Autodesk Inventor part; units mm, degrees
ref_plane "YZ Plane" through (0, 0, 0) normal (1, 0, 0) x (0, 1, 0)
ref_plane "XZ Plane" through (0, 0, 0) normal (0, 1, 0) x (-1, 0, 0)
ref_plane "XY Plane" through (0, 0, 0) normal (0, 0, 1) x (1, 0, 0)
sketch "Szkic1" plane through (0, 0, 0) normal (0, 1, 0) x (-1, 0, 0)
  line L0 (0, 0) -> (-50, 0)
  line L1 (-50, 0) -> (-50, -90)
  line L2 (-50, -90) -> (0, -90)
  line L3 (0, -90) -> (0, 0)
  dimension "d0" = 50
  dimension "d1" = 90
extrude "Wyciągnięcie proste1" add sketch "Szkic1" along normal blind 20
sketch "Szkic2" plane through (0, 20, 0) normal (0, 1, 0) x (1, 0, 0)
  line L0 (50, 0) -> (50, 90)
  line L1 (50, 65) -> (30, 65)
  line L2 (30, 65) -> (30, 25)
  line L3 (30, 25) -> (50, 25)
  line L4 (50, 25) -> (50, 65)
  line L5 (50, 90) -> (0, 90)
  point P0 (0, 0)
  dimension "d4" = 20
  dimension "d5" = 40
  dimension "d6" = 25
extrude "Wyciągnięcie proste2" cut sketch "Szkic2" against normal blind 10
sketch "Szkic3" plane through (0, 10, 0) normal (0, 1, 0) x (1, 0, 0)
  line L0 (50, 65) -> (50, 25)
  circle A0 centre (50, 45) radius 10
  point P0 (0, 0)
  point P1 (50, 35)
  point P2 (50, 55)
  dimension "d9" = 20
extrude "Wyciągnięcie proste3" cut sketch "Szkic3" against normal through all contours L0 A0 picked at (46.1942, 47.495)
sketch "Szkic4" plane through (0, 0, 0) normal (0, -1, 0) x (1, 0, 0)
  line L0 (0, 0) -> (50, 0)
  line L1 (50, -90) -> (0, -90)
  line L2 (15, 0) -> (35, 0)
  line L3 (35, 0) -> (35, -90)
  line L4 (35, -90) -> (15, -90)
  line L5 (15, -90) -> (15, 0)
  line L6 (0, -90) -> (0, 0)
  dimension "d12" = 20
  dimension "d13" = 15
extrude "Wyciągnięcie proste4" cut sketch "Szkic4" against normal blind 5 contours L0 L3 L1 L5
sketch "Szkic5" plane through (0, 0, 0) normal (1, 0, 0) x (0, 1, 0)
  line L0 (20, -65) -> (20, -90)
  line L1 (20, -75) -> (35, -75)
  line L2 (35, -75) -> (50, -55.1735)
  line L3 (50, -55.1735) -> (50, -45.1735)
  line L4 (20, -25) -> (20, -65)
  line L5 (20, -15) -> (35, -15)
  line L6 (35, -15) -> (50, -34.8265)
  line L7 (50, -34.8265) -> (50, -44.8265)
  line L8 (20, -75) -> (20, -15)
  line L9 (20, -90) -> (20, 0)
  line L10 (50, -55.1735) -> (50, -34.8265)
  point P0 (0, 0)
  dimension "d16" = 15
  dimension "d17" = 10
  dimension "d18" = 15
extrude "Wyciągnięcie proste5" add sketch "Szkic5" along normal blind 18
sketch "Szkic6" plane through (18, 0, 0) normal (1, 0, 0) x (0, 0, -1)
  line L0 (25, 20) -> (65, 20)
  line L1 (15, 35) -> (15, 20)
  point P0 (0, 0)
  point P1 (45, 35)
  point P2 (45, 20)
  point P3 (15, 27.5)
  dimension "d21" = 15
  dimension "d22" = 30
hole "Otwór1" at (18, 35, -45) direction (-1, 0, 0) diameter 18 end through all
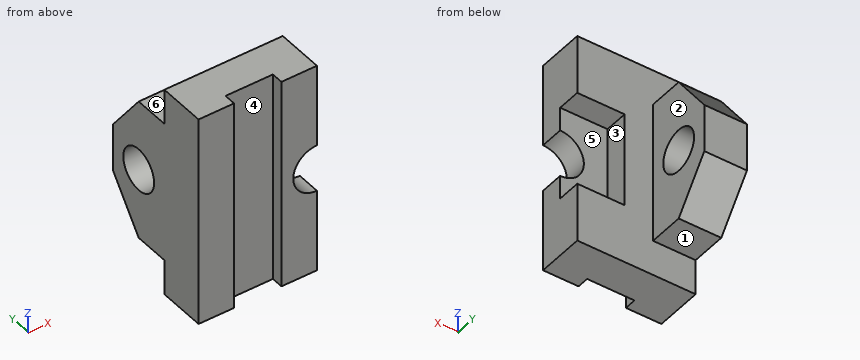
For this review, take the finished solid that the model builds, in its own axes (mm). Face numbers are marked on the shaded views. A direction names the side the tool comes from. Round coordinates to 2 decimals unless told otherwise and drop trailing zeros. Order: outer loops, then holes, each group sorted by start corner. A loop starts at its lowest first (then second) coordinate and runs counter-clockwise, first axis right, second up.
Q1. Insertion check: P1, Ø6, axis at x = 29.5, z = -33.5, coming from the -Y side; P2, Ø22, axis at x = 38, z = -40, coming from the +Y side; P3, Ø8, axis at x = 5.5, y = 26.5, coming from the +Z side. Each pin has a flat end and moves straight along its axis. Give the tip position at first contact, or say it passes through.
Findings below:
P1: stops at y = 5
P2: stops at y = 20
P3: stops at z = -15
Q2. We need section C-C, the plane y = 18.5. Give the boundary of the cut face in (x, z), plus the area to 3 significant figures.
Findings below:
outline: (0, -90) - (50, -90) - (50, -65) - (30, -65) - (30, -25) - (50, -25) - (50, 0) - (0, 0) - close
area: 3,700 mm2
Q3. Machinability: for the marked faces 1, 2 and 3, which of the approach directions +Z, -Z, +X, -X, +Y, -Y give a long, thin tool a straight path to every point of the face, cutting with its end or side? Answer none if there is none.
Findings below:
face 1: -Z, +X, -X, +Y
face 2: +Z, -Z, +X, +Y
face 3: +X, +Y
Q4. We need section A-A, the plane z = -45. Give the boundary of the cut face in (x, y).
Findings below:
outline: (0, 0) - (15, 0) - (15, 5) - (35, 5) - (35, 0) - (40, 0) - (40, 10) - (30, 10) - (30, 20) - (18, 20) - (18, 26) - (0, 26) - close; (0, 44) - (18, 44) - (18, 50) - (0, 50) - close
Q5. Wall thickness on line 1 (Z direction, x = 7.75, y = 35); line 2 (Y direction, x = 14, z = -45); line 3 (X direction, y = 2, z = -70): over which ranges is each line inside the solid? List them lowest first.
Findings below:
line 1: z = -75 to -54, -36 to -15
line 2: y = 0 to 26, 44 to 50
line 3: x = 0 to 15, 35 to 50
Q6. Mouldability with a two-part tool opening along Z and no side actions: class the marked faces 4, 5 and 6 as pulls with the +Z half, pulls with the -Z half, needs draft (parallel to the pull), parting line crosses it, or undercut.
Findings below:
face 4: needs draft
face 5: undercut
face 6: pulls with the +Z half
Q7. We need section D-D, the plane y = 34. Give the boundary of the cut face in (x, z).
Findings below:
outline: (0, -75) - (18, -75) - (18, -53.94) - (0, -53.94) - close; (0, -36.06) - (18, -36.06) - (18, -15) - (0, -15) - close
Q8. We need section B-B, the plane x = 8. Give the boundary of the cut face in (y, z), plus the area to 3 significant figures.
Findings below:
outline: (0, -90) - (20, -90) - (20, -75) - (35, -75) - (50, -55.17) - (50, -34.83) - (35, -15) - (20, -15) - (20, 0) - (0, 0) - close; hole circle Ø18 at (35, -45)
area: 3,050 mm2
